```python
from build123d import *

# Parameters (mm, degrees)
BOSS_EXTRUDE1_DEPTH     = 12.7
CUT_EXTRUDE1_DEPTH      = 28.189075625
CUT_EXTRUDE1_DEPTH_BACK = 28.189075625
SKETCH2_R               = 2.54


with BuildPart() as part:
    # Sketch1 → Boss-Extrude1 (new, symmetric)
    with BuildSketch(Plane.XY):
        Polygon((6.35, 3.666174209), (0, 7.332348419), (-6.35, 3.666174209), (-6.35, -3.666174209), (0, -7.332348419), (6.35, -3.666174209), align=None)
    extrude(amount=BOSS_EXTRUDE1_DEPTH, both=True)

    # Sketch2 → Cut-Extrude1 (cut, two sides: drawn at the far end of the back side and taken through both)
    with BuildSketch(Plane.XY.offset(12.7).offset(-CUT_EXTRUDE1_DEPTH_BACK)):
        Circle(SKETCH2_R)
    extrude(amount=CUT_EXTRUDE1_DEPTH + CUT_EXTRUDE1_DEPTH_BACK, mode=Mode.SUBTRACT)


solid = part.part
```
Source: CAD feature listing. Evaluate the final solid. Frame: model axes, mm. Round coordinates to 2 decimals unless told otherwise and drop trailing zeros. Loops run counter-clockwise (first coordinate to the right, second up) from the corner with the lowest first, then second, coordinate; pieces in that order, holes last. Notation, with made-up numbers: M 32.25,51 L 37.25,51 A7 cw 37.25,59 Z; hole C 78,79.5 d7. An arc over 180 degrees is marked long. Use a Markdown table: item, result. Add a question column.
1. Contact query for a flat-ended pin moving along its axis: pin 1 (3 mm diameter, centred on x = -3, z = 0.5, fed in from +Y). Output: stop coordinate, or through.
2. Pull-direction query (X, two-part tool) for faces 1 (the flat face through (0, -3, -12.7)), 2 (the cylindrical face through (-0.33, 2.52, -0.18)), 3 (the flat face through (3.131, -5.525, 0.178)); classes: +X half, -X half, draft (parallel to the pull), parting line (faces both ways), or undercut.
3. Cut plane D-D, the plane y = 4. Output: boundary loops of the cut face in (x, z).
4. Cut plane A-A, the plane y = 0. Output: boundary loops of the cut face in (x, z).
5. Cut plane B-B, the plane z = 7.75. Output: boundary loops of the cut face in (x, y).
6. Ray query, line 1 along X through (y, z) = (0, 4.75); line 2 along X through (y, z) = (1, -0.5); line 3 along Y through (x, z) = (4.5, 8). Return the intervals inside material, ascending. Write a range as [from, to].
7. Cut plane C-C, the plane x = 0.75. Output: boundary loops of the cut face in (y, z).
Solution:
| question | item | result |
|---|---|---|
| 1 | pin 1 | stops at y = 6.47 |
| 2 | face 1 | draft |
| 2 | face 2 | undercut |
| 2 | face 3 | +X half |
| 3 | outline | M -5.77,-12.7 L 5.77,-12.7 L 5.77,12.7 L -5.77,12.7 Z |
| 4 | outline | M -6.35,-12.7 L -2.54,-12.7 L -2.54,12.7 L -6.35,12.7 Z; M 2.54,-12.7 L 6.35,-12.7 L 6.35,12.7 L 2.54,12.7 Z |
| 5 | outline | M -6.35,-3.67 L 0,-7.33 L 6.35,-3.67 L 6.35,3.67 L 0,7.33 L -6.35,3.67 Z; hole C 0,0 d5.08 |
| 6 | line 1 | x = [-6.35, -2.54], [2.54, 6.35] |
| 6 | line 2 | x = [-6.35, -2.33], [2.33, 6.35] |
| 6 | line 3 | y = [-4.73, 4.73] |
| 7 | outline | M -6.9,-12.7 L -2.43,-12.7 L -2.43,12.7 L -6.9,12.7 Z; M 2.43,-12.7 L 6.9,-12.7 L 6.9,12.7 L 2.43,12.7 Z |
